Design review of the part built by this model. Coordinates are the model's own, in mm. Face numbers are marked on the shaded views. Give positions to 0.01 mm unless a question says otherwise; leave off trailing zeros. Loops run counter-clockwise (first coordinate to the right, second up) from the corner with the lowest first, then second, coordinate; pieces in that order, holes last. Notation, with made-up numbers: M 26,-20 L 65,-20 A31 ccw 65,12 Z; hole C 57,30 d8. An arc over 180 degrees is marked long. Answer as CSV lines item,"result".
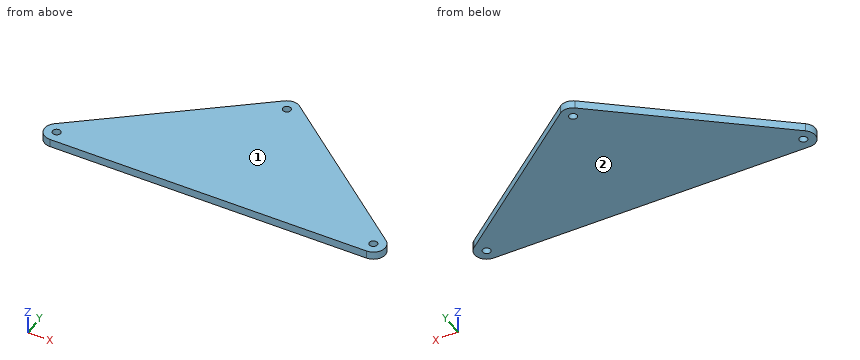
```python
from build123d import *

# Parameters (mm, degrees)
SKETCH1_R           = 4.7625
SKETCH1_R_2         = 1.5875
BOSS_EXTRUDE1_DEPTH = 3.175


with BuildPart() as part:
    # Sketch1 → Boss-Extrude1 (new body)
    # profile 1 of 4: a face of its own
    with BuildSketch(Plane.XY):
        with BuildLine():
            ThreePointArc((68.2625, 50.8), (61.436938671, 46.507543337), (60.524889836, 54.518887705))
            Line((60.524889836, 54.518887705), (-2.975110164, 3.718887705))
            ThreePointArc((-2.975110164, 3.718887705), (2.063061329, 4.292456663), (4.7625, 0))
            ThreePointArc((4.7625, 0), (3.367596045, -3.367596045), (0, -4.7625))
            Line((0, -4.7625), (127, -4.7625))
            ThreePointArc((127, -4.7625), (122.50597013, 1.576420559), (129.975110164, 3.718887705))
            Line((129.975110164, 3.718887705), (66.475110164, 54.518887705))
            ThreePointArc((66.475110164, 54.518887705), (67.792456663, 52.863061329), (68.2625, 50.8))
        make_face()
    # profile 2 of 4: a face of its own
    with BuildSketch(Plane.XY):
        Circle(SKETCH1_R)
        with Locations(Location((0, 0, 0), (0, 0, 180))):
            Circle(SKETCH1_R_2, mode=Mode.SUBTRACT)
    # profile 3 of 4: a face of its own
    with BuildSketch(Plane.XY):
        with Locations((63.5, 50.8)):
            Circle(SKETCH1_R)
        with Locations(Location((63.5, 50.8, 0), (0, 0, 180))):
            Circle(SKETCH1_R_2, mode=Mode.SUBTRACT)
    # profile 4 of 4: a face of its own
    with BuildSketch(Plane.XY):
        with Locations((127, 0)):
            Circle(SKETCH1_R)
        with Locations(Location((127, 0, 0), (0, 0, 180))):
            Circle(SKETCH1_R_2, mode=Mode.SUBTRACT)
    extrude(amount=BOSS_EXTRUDE1_DEPTH)


solid = part.part
```
1. For P1, Ø4, axis at x = 127, y = 0, coming from the +Z side (3 decimals); P2, Ø1.5, axis at y = 26.5, z = 0.5, coming from the -X side; P3, Ø1, axis at y = 4.5, z = 2.5, coming from the -X side, all flat-tipped, find the tip position at first contact; note any pin that passes through.
Answer block:
P1,"z = 3.175"
P2,"x = 24.56"
P3,"x = -2.62"
2. We need section A-A, the plane y = 0. Write out the cut boundary in (x, z) (1 decimal), plus the area to 3 significant figures.
Answer block:
outline,"M -4.8,0 L -1.6,0 L -1.6,3.2 L -4.8,3.2 Z; M 1.6,0 L 125.4,0 L 125.4,3.2 L 1.6,3.2 Z; M 128.6,0 L 131.8,0 L 131.8,3.2 L 128.6,3.2 Z"
area,"413 mm²"
3. To check wall thickness, follow L1, parallel to X at y = 50.8, z = 2.45; L2, parallel to Y at x = 127, z = 2.15; L3, parallel to Y at x = 42, z = 1.15. State the ranges of each line that lie inside material, in increasing order. Write a range as [from, to].
Answer block:
L1,"[55.88, 61.91], [65.09, 71.12]"
L2,"[-4.76, -1.59], [1.59, 6.1]"
L3,"[-4.76, 39.7]"
4. We need section C-C, the plane y = 50.8. Write out the cut boundary in (x, z) (1 decimal).
Answer block:
outline,"M 55.9,0 L 61.9,0 L 61.9,3.2 L 55.9,3.2 Z; M 65.1,0 L 71.1,0 L 71.1,3.2 L 65.1,3.2 Z"
5. We need section D-D, the plane x = 20. Write out the cut boundary in (y, z) (1 decimal), plus the area to 3 significant figures.
Answer block:
outline,"M -4.8,0 L 22.1,0 L 22.1,3.2 L -4.8,3.2 Z"
area,"85.3 mm²"
6. The part is to be moulded in two halves that separate along Z. For the marked faces 1 and 2, say which applies: pulls with the +Z half, pulls with the -Z half, needs draft (parallel to the pull), parting line crosses it, or undercut.
Answer block:
face 1,"pulls with the +Z half"
face 2,"pulls with the -Z half"
7. We need section B-B, the plane z = 0.5. Write out the cut boundary in (x, y) (1 decimal), plus the area to 3 significant figures.
Answer block:
outline,"M -3,3.7 A4.8 ccw 0,-4.8 L 127,-4.8 A4.8 ccw 130,3.7 L 66.5,54.5 A4.8 ccw 60.5,54.5 Z; hole C 0,0 d3.2; hole C 63.5,50.8 d3.2; hole C 127,0 d3.2"
area,"4,650 mm²"
